Build history of the part. All positions in model axes, mm. Round coordinates to 2 decimals unless told otherwise and drop trailing zeros. Write each loop counter-clockwise with the first axis right and the second up, starting at its lowest first coordinate (ties: lowest second). Pieces come first, ordered by that corner, then holes. Notation, with made-up numbers: (58, -8.75) - (110, -8.75) arc R23 cw to (110, 10.25) - close; hole circle Ø1 at (49, 43). An arc over 180 degrees is marked (long way). Write each question's results on one line, items separated by ' | '.
from build123d import *

# Parameters (mm, degrees)
BOSS_EXTRUDE1_DEPTH     = 2032
SKETCH2_W               = 211.702458594
SKETCH2_H               = 483.586926944
CUT_EXTRUDE1_DEPTH      = 50
SKETCH3_W               = 200.611820878
SKETCH3_H               = 857.421683483
CUT_EXTRUDE3_DEPTH      = 85.870489571
CUT_EXTRUDE3_DEPTH_BACK = 2.54


with BuildPart() as part:
    # Sketch1 → Boss-Extrude1 (new body)
    with BuildSketch(Plane.XY):
        with BuildLine():
            Line((-27.5, 49), (27.5, 49))
            Line((27.5, 49), (27.5, 44.3))
            Line((27.5, 44.3), (8.8, 44.3))
            ThreePointArc((8.8, 44.3), (3.850252532, 42.249747468), (1.8, 37.3))
            Line((1.8, 37.3), (1.8, -37.3))
            ThreePointArc((1.8, -37.3), (3.850252532, -42.249747468), (8.8, -44.3))
            Line((8.8, -44.3), (27.5, -44.3))
            Line((27.5, -44.3), (27.5, -49))
            Line((27.5, -49), (-27.5, -49))
            Line((-27.5, -49), (-27.5, -44.3))
            Line((-27.5, -44.3), (-8.8, -44.3))
            ThreePointArc((-8.8, -44.3), (-3.850252532, -42.249747468), (-1.8, -37.3))
            Line((-1.8, -37.3), (-1.8, 37.3))
            ThreePointArc((-1.8, 37.3), (-3.850252532, 42.249747468), (-8.8, 44.3))
            Line((-8.8, 44.3), (-27.5, 44.3))
            Line((-27.5, 44.3), (-27.5, 49))
        make_face()
    extrude(amount=BOSS_EXTRUDE1_DEPTH)

    # Sketch2 → Cut-Extrude1 (cut, through all)
    with BuildSketch(Plane(origin=(0, -12.25, 21.217622393), x_dir=(1, 0, 0), z_dir=(0, -0.5, 0.866025404))):
        with Locations((0, 13.030857736)):
            Rectangle(SKETCH2_W, SKETCH2_H)
    extrude(amount=-CUT_EXTRUDE1_DEPTH, mode=Mode.SUBTRACT)

    # Sketch3 → Cut-Extrude3 (cut, two sides)
    with BuildSketch(Plane(origin=(0, 843.131810245, 486.782377607), x_dir=(1, 0, 0), z_dir=(0, 0.866025404, 0.5))) as cut_extrude3_sk:
        with Locations((6.979656851, -1512.870182956)):
            Rectangle(SKETCH3_W, SKETCH3_H)
    extrude(amount=CUT_EXTRUDE3_DEPTH, mode=Mode.SUBTRACT)
    extrude(cut_extrude3_sk.sketch, amount=-CUT_EXTRUDE3_DEPTH_BACK, mode=Mode.SUBTRACT)


solid = part.part
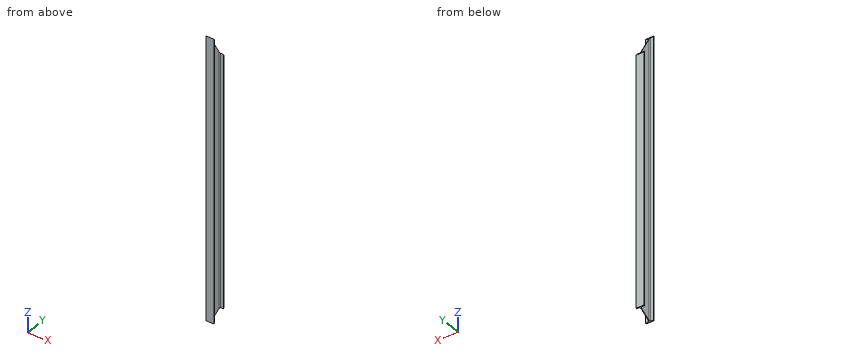
(1) Flat gauge pins, fed straight in: pin 1 Ø6 at (y, z) = (-34.5, 559.5) entering from -X; pin 2 Ø5 at (y, z) = (-13, 302.5) entering from +X; pin 3 Ø12 at (x, y) = (-6, -11) entering from -Z. Where does each tip first touch, or does it go through?
Worked answers:
pin 1: stops at x = -1.8 | pin 2: stops at x = 1.8 | pin 3: stops at z = 19.47
(2) Drill centre lines: probe 1 along Y at (x, z) = (21, 688.5); probe 2 along Y at (x, z) = (-6.5, 1591.5); probe 3 along X at (y, z) = (-10, 1603). Where is each one in solid material? Low to high. Write a range as [from, to].
Worked answers:
probe 1: y = [-49, -44.3], [44.3, 49] | probe 2: y = [-49, -43.91], [43.91, 49] | probe 3: x = [-1.8, 1.8]
(3) Slice it at B-B, the plane y = 22. Write the cut outline in (x, z), and give its area (3 significant figures).
Worked answers:
outline: (-1.8, 40.99) - (1.8, 40.99) - (1.8, 1903.94) - (-1.8, 1903.94) - close | area: 6,710 mm2
(4) Slice it at A-A, the plane z = 668. Write the cut outline in (x, y), and give its area (3 significant figures).
Worked answers:
outline: (-27.5, -49) - (27.5, -49) - (27.5, -44.3) - (8.8, -44.3) arc R7 cw to (1.8, -37.3) - (1.8, 37.3) arc R7 cw to (8.8, 44.3) - (27.5, 44.3) - (27.5, 49) - (-27.5, 49) - (-27.5, 44.3) - (-8.8, 44.3) arc R7 cw to (-1.8, 37.3) - (-1.8, -37.3) arc R7 cw to (-8.8, -44.3) - (-27.5, -44.3) - close | area: 878 mm2
